```python
from build123d import *

# Parameters (mm, degrees)
F0_R     = 4.5
F0_R_2   = 3.5
F1_DEPTH = 11
F2_W     = 3.2331479252
F2_H     = 2
F3_DEPTH = 8
F4_R     = 6
F5_DEPTH = 16
F6_SIZE2 = 1.49999
F6_SIZE  = 3.99999
F8_DEPTH = 10


# Not quite as in the source:
# - a fillet or chamfer is up to 0.001 mm smaller than in the source, because OpenCascade refuses the exact size


with BuildPart() as f1:
    # F0 (on Top) → F1 (new body)
    with BuildSketch(Plane.XY):
        Circle(F0_R)
        Circle(F0_R_2, mode=Mode.SUBTRACT)
    extrude(amount=F1_DEPTH)

    # F2 (on face) → F3 (join)
    with BuildSketch(Plane.XY.offset(11)):
        with Locations((-5.2334260374, 0)):
            Rectangle(F2_W, F2_H)
        with Locations((5.2334260374, 0)):
            Rectangle(F2_W, F2_H)
    extrude(amount=-F3_DEPTH)

    # F4 (on face) → F5 (join)
    with BuildSketch(Plane(origin=(0, 0, 0), x_dir=(1, 0, 0), z_dir=(0, 0, -1))):
        Circle(F4_R)
    extrude(amount=F5_DEPTH)

    # F6 (size 4 and 1.5 in the source; OpenCascade refuses exactly that, so slightly less here)
    f6_edges = [f1.edges().sort_by_distance(p)[0] for p in [
        (-6, 0, 0),
    ]]
    f6_side = f1.faces().sort_by_distance((-6, 0, -8))[0]
    chamfer(f6_edges, length=F6_SIZE, length2=F6_SIZE2, reference=f6_side)

    # F7 (on face) → F8 (cut)
    with BuildSketch(Plane(origin=(0, 0, -16), x_dir=(1, 0, 0), z_dir=(0, 0, -1))):
        Polygon((-1.5, 1.5), (-4, 1.5), (-4, -1.5), (-1.5, -1.5), (-1.5, -4), (1.5, -4), (1.5, -1.5), (4, -1.5), (4, 1.5), (1.5, 1.5), (1.5, 4), (-1.5, 4), align=None)
    extrude(amount=-F8_DEPTH, mode=Mode.SUBTRACT)


solid = f1.part
```
The listing builds one solid part. Answer for the finished solid, in the listing's coordinates (mm). A direction names the side the tool comes from. Give positions to 0.01 mm unless a question says otherwise; leave off trailing zeros. Order: outer loops, then holes, each group sorted by start corner. A loop starts at its lowest first (then second) coordinate and runs counter-clockwise, first axis right, second up. Notation, with made-up numbers: (27.5, -13.5) - (84.5, -13.5) arc R20 ccw to (84.5, 16.5) - close; hole circle Ø10 at (-3.75, -29). An arc over 180 degrees is marked (long way). Answer in a Markdown table with one row per item. Add a question column.
Q1. The part is cut by section D-D (z = -6.5). Determine the outline of the cut face in (x, y).
Q2. Which of the six approach directions +Z, -Z, +X, -X, +Y, -Y give full straight-line access (tool end or side, diameter ignored) to faces 1 (the flat face through (3, -1.5, -11)), 2 (the cylindrical face through (3.233, -1.341, 5.423)), 3 (the flat face through (6, 1, 7))?
Q3. The part is cut by section A-A (z = 6.75). Determine the outline of the cut face in (x, y).
Q4. Given P1, Ø1.5, axis at x = -5, z = -4, coming from the +Y side; P2, Ø2.5, axis at x = 6, z = 6, coming from the +Y side; P3, Ø3.5, axis at y = -0.5, z = -10.5, coming from the +X side, each flat-ended and moving along its own axis, determine where each tip first touches the part or whether it passes through.
Q5. Find the intervals of material crossed by line 1 along Y through (x, z) = (0, 8.5); line 2 along Z through (x, y) = (-2, 1.25); line 3 along X through (y, z) = (2.75, -10.5), in increasing order. Write a range as [from, to].
Q6. For a pull along Z with two mould halves and no side action, classify faces 4 (the flat face through (-6, 0, 3)), 5 (the flat face through (-6, 1, 7)), 6 (the flat face through (-4, 0, 11)) as released by +Z, released by -Z, zero draft, split by the parting line, or undercut.
Determined:
| question | item | result |
|---|---|---|
| 1 | outline | circle Ø12 at (0, 0); hole (-4, -1.5) - (-1.5, -1.5) - (-1.5, -4) - (1.5, -4) - (1.5, -1.5) - (4, -1.5) - (4, 1.5) - (1.5, 1.5) - (1.5, 4) - (-1.5, 4) - (-1.5, 1.5) - (-4, 1.5) - close |
| 2 | face 1 | -Z |
| 2 | face 2 | +Z |
| 2 | face 3 | +Z, +X, +Y |
| 3 | outline | (-6.85, -1) - (-4.39, -1) arc R4.5 ccw to (4.39, -1) - (6.85, -1) - (6.85, 1) - (4.39, 1) arc R4.5 ccw to (-4.39, 1) - (-6.85, 1) - close; hole circle Ø7 at (0, 0) |
| 4 | P1 | stops at y = 4.24 |
| 4 | P2 | stops at y = 1 |
| 4 | P3 | stops at x = 6 |
| 5 | line 1 | y = [-4.5, -3.5], [3.5, 4.5] |
| 5 | line 2 | z = [-6, 0] |
| 5 | line 3 | x = [-5.33, -1.5], [1.5, 5.33] |
| 6 | face 4 | undercut |
| 6 | face 5 | zero draft |
| 6 | face 6 | released by +Z |
